Autodesk Inventor part; units mm, degrees
ref_plane "YZ Plane" through (0, 0, 0) normal (1, 0, 0) x (0, 1, 0)
ref_plane "XZ Plane" through (0, 0, 0) normal (0, 1, 0) x (-1, 0, 0)
ref_plane "XY Plane" through (0, 0, 0) normal (0, 0, 1) x (1, 0, 0)
sketch "Esquisse1" plane through (0, 0, 0) normal (0, 1, 0) x (-1, 0, 0)
  line L0 (14.0671, 6.9597) -> (-17.9329, 6.9597)
  line L1 (-17.9329, 6.9597) -> (-17.9329, -18.0403)
  line L2 (-17.9329, -18.0403) -> (14.0671, -18.0403)
  line L3 (14.0671, -18.0403) -> (14.0671, 6.9597)
  point P0 (0, 0)
  dimension "d0" = 25
  dimension "d1" = 32
extrude "Extrusion1" add sketch "Esquisse1" along normal blind 30
sketch "Esquisse2" plane through (0, 30, 0) normal (0, 1, 0) x (1, 0, 0)
  circle A0 centre (1.9329, 9.0403) radius 15
  line L0 (-14.0671, 18.0403) -> (-14.0671, -6.9597)
  line L1 (-14.0671, -6.9597) -> (17.9329, -6.9597)
  point P0 (0, 0)
  dimension "d4" = 30
  dimension "d5" = 16
  dimension "d6" = 16
extrude "Extrusion2" cut sketch "Esquisse2" against normal blind 28
sketch "Esquisse3" plane through (1.9329, 2, -9.0403) normal (0, 1, 0) x (1, 0, 0)
  circle A0 centre (0, 0) radius 5
  line L0 (16, 9) -> (-16, 9)
  line L1 (-16, 9) -> (-16, -16)
  line L2 (-16, -16) -> (16, -16)
  point P0 (-1.9329, -9.0403)
  dimension "d9" = 10
  dimension "d11" = 16
  dimension "d14" = 16
extrude "Extrusion3" cut sketch "Esquisse3" against normal through all
sketch "Esquisse5" plane through (17.9329, 0, -18.0403) normal (0, 0, -1) x (-1, 0, 0)
  line L0 (28, 30) -> (28, 2)
  line L1 (32, 30) -> (28, 30)
  line L2 (28, 30) -> (28, 16)
  line L3 (28, 16) -> (32, 16)
  line L4 (32, 16) -> (32, 30)
  line L5 (28, 30) -> (32, 30)
  line L6 (32, 0) -> (32, 30)
  line L7 (4, 2) -> (4, 30)
  line L8 (0, 30) -> (4, 30)
  line L9 (4, 16) -> (0, 16)
  line L10 (0, 16) -> (0, 30)
  line L11 (0, 30) -> (4, 30)
  line L12 (4, 30) -> (4, 16)
  point P0 (17.9329, 0)
  dimension "d15" = 14
  dimension "d16" = 0
  dimension "d17" = 0
  dimension "d18" = 14
extrude "Extrusion4" add sketch "Esquisse5" along normal blind 10
sketch "Esquisse6" plane through (17.9329, 0, -28.0403) normal (0, 0, -1) x (-1, 0, 0)
  line L0 (32, 16) -> (28, 16)
  line L1 (32, 30) -> (0, 30)
  line L2 (32, 16) -> (0, 16)
  line L3 (0, 16) -> (0, 30)
  line L4 (0, 30) -> (32, 30)
  line L5 (32, 30) -> (32, 16)
  point P0 (17.9329, 0)
extrude "Extrusion5" add sketch "Esquisse6" along normal blind 50
sketch "Esquisse7" plane through (17.9329, 0, -78.0403) normal (0, 0, -1) x (-1, 0, 0)
  line L0 (32, 30) -> (0, 30)
  line L1 (32, 30) -> (0, 30)
  line L2 (0, 30) -> (0, -30)
  line L3 (0, -30) -> (32, -30)
  line L4 (32, -30) -> (32, 30)
  point P0 (17.9329, 0)
  dimension "d23" = 60
extrude "Extrusion6" add sketch "Esquisse7" along normal blind 10
sketch "Esquisse8" plane through (17.9329, 0, 6.9597) normal (1, 0, 0) x (0, 0, -1)
  ellipse E0 centre (54.9571, -14.73) end of major axis (54.9571, -44.73) minor radius 29.9996
  ellipse E1 centre (54.9571, -14.73) end of major axis (54.9571, 12.27) minor radius 26.9996
  ellipse E2 centre (54.9571, -14.73) end of major axis (54.9571, -44.73) minor radius 29.9996
  arc A0 (82.092, -27.5236) -> (27.8222, -1.9363) centre (54.9571, -14.73) ccw
  line L0 (85, 16) -> (85, -30)
  line L1 (82.092, -27.5236) -> (85, -30)
  line L2 (25, 16) -> (85, 16)
  line L3 (85, -30) -> (85, 16)
  line L4 (85, 16) -> (25, 16)
  line L5 (25, 0) -> (25, 16)
  line L6 (25, 16) -> (25, 0)
  line L7 (25, 0) -> (27.8222, -1.9363)
  point P0 (6.9597, 0)
extrude "Extrusion7" add sketch "Esquisse8" against normal blind 32 contours E0 L7 L5 L2 L0 L1
fillet "Congé1" radius 30 1 edges at (1.9329, 30, -88.0403)
fillet "Congé2" radius 10 1 edges at (1.9329, -30, -88.0403)
sketch "Esquisse9" plane through (-10.0671, 16, -28.0403) normal (0, 1, 0) x (1, 0, 0)
  circle A0 centre (12, -19) radius 5
  line L0 (0, -10) -> (24, -10)
  arc A1 (0, -10) -> (24, -10) centre (12, -19) ccw
  circle A2 centre (12, -19) radius 15
  point P0 (10.0671, -28.0403)
  dimension "d30" = 30
extrude "Extrusion8" cut sketch "Esquisse9" against normal up to surface (14 mm away) contours A2 L0
sketch "Esquisse10" plane through (-14.0671, 0, 6.9597) normal (0, 0, 1) x (1, 0, 0)
  line L0 (32, 15.27) -> (32, -27.5236)
  line L1 (0, 30) -> (32, 30)
  line L2 (32, 30) -> (32, 0)
  line L3 (32, 0) -> (0, 0)
  line L4 (0, 0) -> (0, 30)
  point P0 (14.0671, 0)
  point P1 (32, -1.9363)
extrude "Extrusion9" add sketch "Esquisse10" along normal blind 5
sketch "Esquisse11" plane through (0, 30, 0) normal (0, 1, 0) x (1, 0, 0)
  circle A0 centre (1.3437, 52.0208) radius 1.5
  point P0 (0, 0)
extrude "Extrusion10" cut sketch "Esquisse11" against normal through all
properties part number "support-moteur"
Check sheet for the modelled part. Datum: model origin and axes. Units: mm. A direction names the side the tool comes from. Coordinates: 2 decimals unless noted, no trailing zeros. Order: outer loops, then holes, each group sorted by start corner. A loop starts at its lowest first (then second) coordinate and runs counter-clockwise, first axis right, second up. Notation, with made-up numbers: M -30.75,71 L 28.25,71 A27 ccw 28.25,105 Z; hole C 50,50 d7. An arc over 180 degrees is marked long. One line per question, with ' | ' between items. Start each with the question number.
Item 1: Access from +Z, -Z, +X, -X, +Y, -Y to the whole of each face (thin tool, end or side, straight path). Record for faces 1 (the cylindrical face through (2.157, 20.979, -79.485)), 2 (the flat face through (13.933, 23, -23)), 3 (the flat face through (2, 0, -3)).
Item 2: Sectioned sample at A-A on z = -11. Record the cut outline in (x, y).
Item 3: Material ranges on line 1 (Z direction, x = 4, y = 8.5); line 2 (Z direction, x = 7.5, y = 11.5); line 3 (Z direction, x = 5.5, y = -14.5), recorded low to high.
Item 4: Mould release check, pull along Z, two halves, no side actions. Record for faces 4 (the flat face through (2, 30, -31)), 5 (the flat face through (2.157, -0.955, -19.432)), 6 (the cylindrical face through (1.019, 22.485, -50.556)): pulls with the +Z half, pulls with the -Z half, needs draft (parallel to the pull), parting line crosses it, or undercut.
Item 5: Sectioned sample at B-B on y = 20. Record the cut outline in (x, z).
Item 6: Gauge pin test, flat ends, axial feed: P1, Ø5, axis at x = 1.34, z = -52.02, coming from the -Y side; P2, Ø2, axis at x = 2.5, y = -4.5, coming from the +Z side; P3, Ø10, axis at y = -5.5, z = -76.5, coming from the +X side; P4, Ø10, axis at x = 10.5, y = 19, coming from the -Z side. Record the tip position at first contact, or that the pin passes through.
Item 7: Sectioned sample at C-C on y = 8. Count the separate pieces of the cut face and the enclosed holes in it, and give its area (3 significant figures).
Answer below:
1) face 1: -Z, +X, -X, +Y | face 2: +Y | face 3: +Z, +X, -X, -Y
2) outline: M -14.07,0 L -2.67,0 L -2.67,2 L -12.94,2 L -12.94,30 L -14.07,30 Z; M 6.53,0 L 17.93,0 L 17.93,30 L 16.8,30 L 16.8,2 L 6.53,2 Z
3) line 1: z = -86.81 to -66.98, -29.01 to -23.9, 5.82 to 11.96 | line 2: z = -85.75 to -62.56, -33.44 to -22.97, 4.89 to 11.96 | line 3: z = -88.04 to -78
4) face 4: needs draft | face 5: pulls with the +Z half | face 6: undercut
5) outline: M -14.07,-80.4 L 17.93,-80.4 L 17.93,11.96 L -14.07,11.96 Z; hole M -10.07,-28.04 L 13.93,-28.04 L 13.93,-18.04 A15 ccw long -10.07,-18.04 Z; hole C 1.34,-52.02 d3
6) P1: stops at y = 14.55 | P2: stops at z = -75.82 | P3: stops at x = 17.93 | P4: stops at z = -84.57
7) separate pieces: 2 | enclosed holes: 1 | area: 1,210 mm^2
